Read the model definition and answer for the solid it produces. Units are mm, in the model's axes. A direction names the side the tool comes from. Round coordinates to 2 decimals unless told otherwise and drop trailing zeros. Write each loop counter-clockwise with the first axis right and the second up, starting at its lowest first coordinate (ties: lowest second). Pieces come first, ordered by that corner, then holes.
from build123d import *

# Parameters (mm, degrees)
BOSS_EXTRUDE1_DEPTH  = 10
LPATTERN2_COUNT      = 2
LPATTERN2_PITCH      = 78
LPATTERN2_COUNT_DIR2 = 2
LPATTERN2_PITCH_DIR2 = 26
LPATTERN3_COUNT      = 2
LPATTERN3_PITCH      = 20
LPATTERN3_COUNT_DIR2 = 2
LPATTERN3_PITCH_DIR2 = 17


with BuildPart() as part:
    # Sketch1 → Boss-Extrude1 (new body)
    with BuildSketch(Plane.XY):
        Polygon((92.000001103, 39.239999717), (91.240001103, 39.999999717), (1.760001103, 39.999999717), (1.000001103, 39.239999717), (1.000001103, 2.759999717), (1.760001103, 1.999999717), (91.240001103, 1.999999717), (92.000001103, 2.759999717), align=None)
    extrude(amount=BOSS_EXTRUDE1_DEPTH)

    # Sketch4 → CBORE for M6 SHCS1 (revolve, cut)
    with BuildSketch(Plane(origin=(7.500001103, 33.999999717, 10), x_dir=(0, -1, 0), z_dir=(1, 0, 0))):
        Polygon((0, 0), (0, 10), (3.3, 10), (3.3, 6), (5.5, 6), (5.5, 0.025), (5.525, 0), align=None)
    cbore_for_m6_shcs1 = revolve(axis=Axis((7.500001103, 33.999999717, 16.35), (0, 0, -1)), mode=Mode.SUBTRACT)

    # LPattern2: CBORE for M6 SHCS1 2 × 2
    with Locations(*[(i * LPATTERN2_PITCH, -j * LPATTERN2_PITCH_DIR2, 0) for i in range(LPATTERN2_COUNT) for j in range(LPATTERN2_COUNT_DIR2) if (i, j) != (0, 0)]):
        add(cbore_for_m6_shcs1, mode=Mode.SUBTRACT)

    # Sketch6 → CBORE for M4 SHCS1 (revolve, cut)
    with BuildSketch(Plane(origin=(57.000001103, 11.999999717, 0), x_dir=(0, 1, 0), z_dir=(1, 0, 0))):
        Polygon((0, 0), (0, 10), (2.25, 10), (2.25, 4), (4, 4), (4, 0.025), (4.025, 0), align=None)
    cbore_for_m4_shcs1 = revolve(axis=Axis((57.000001103, 11.999999717, -6.35), (0, 0, 1)), mode=Mode.SUBTRACT)

    # LPattern3: CBORE for M4 SHCS1 2 × 2
    with Locations(*[(-i * LPATTERN3_PITCH, j * LPATTERN3_PITCH_DIR2, 0) for i in range(LPATTERN3_COUNT) for j in range(LPATTERN3_COUNT_DIR2) if (i, j) != (0, 0)]):
        add(cbore_for_m4_shcs1, mode=Mode.SUBTRACT)


solid = part.part
Q1. Straight lines are drawn through the part: probe 1 along X at (y, z) = (34, 6.5); probe 2 along X at (y, z) = (12, 0.95); probe 3 along X at (y, z) = (11, 7). For each, find the intervals that lie inside material, in ascending order.
Verdict:
probe 1: x = 1 to 2, 13 to 80, 91 to 92
probe 2: x = 1 to 33, 41 to 53, 61 to 92
probe 3: x = 1 to 2.89, 12.11 to 34.98, 39.02 to 54.98, 59.02 to 80.89, 90.11 to 92
Q2. Section B-B (y = 34) is taken. Determine the outline of the cut face in (x, z) (3 decimals), then the cut area to 3 significant figures.
Verdict:
outline: (1, 0) - (4.2, 0) - (4.2, 4) - (2, 4) - (2, 9.975) - (1.975, 10) - (1, 10) - close; (10.8, 0) - (82.2, 0) - (82.2, 4) - (80, 4) - (80, 9.975) - (79.975, 10) - (13.025, 10) - (13, 9.975) - (13, 4) - (10.8, 4) - close; (88.8, 0) - (92, 0) - (92, 10) - (91.025, 10) - (91, 9.975) - (91, 4) - (88.8, 4) - close
area: 725 mm2
Q3. Which of the six approach directions +Z, -Z, +X, -X, +Y, -Y give full straight-line access (tool end or side, diameter ignored) to faces 4 (the flat face through (85, 38, 4)), 5 (the cylindrical face through (86.76, 30.95, 2.03)), 6 (the cylindrical face through (40.549, 13.846, 1.985))?
Verdict:
face 4: +Z
face 5: +Z, -Z
face 6: -Z
Q4. Flat-ended cylindrical pins translate along their axes: pin 1 Ø5 at (x, y) = (37, 29) entering from -Z; pin 2 Ø10.5 at (x, y) = (7.5, 34) entering from +Z; pin 3 Ø3.5 at (x, y) = (6.5, 33) entering from +Z. Find the tip coordinate at first contact, or state that the pin passes through.
Verdict:
pin 1: stops at z = 4
pin 2: stops at z = 4
pin 3: passes through
Q5. Determine the mould class of faces 1 (the flat face through (7, 38, 4)), 2 (the flat face through (46, 21, 0)), 3 (the flat face through (47, 40, 5)) for opening direction Y: pulls with the +Y half, pulls with the -Y half, needs draft (parallel to the pull), parting line crosses it, or undercut.
Verdict:
face 1: undercut
face 2: needs draft
face 3: pulls with the +Y half
Q6. Section A-A (z = 6.25) is taken. State how many separate pieces and enclosed holes the cut face has, then the cut area to 3 significant figures.
Verdict:
separate pieces: 1
enclosed holes: 8
area: 3,010 mm2
